Geometry check sheet. Reference: the model listing, model coordinates, mm. Face numbers are marked on the shaded views. A direction names the side the tool comes from. Give positions to 0.01 mm unless a question says otherwise; leave off trailing zeros. Put each result on its own line as item: value. Start each with the question number.
Q1. Go/stop test with flat-tipped pins: pin 1 (2 mm diameter, centred on y = -6.5, z = 1, fed in from -X); pin 2 (9.5 mm diameter, centred on y = -3, z = 37, fed in from -X); pin 3 (5 mm diameter, centred on x = 19, z = 4, fed in from -Y) (3 decimals). Record where each tip stops, or that it passes through.
Q2. Mould release check, pull along Y, two halves, no side actions. Record for the marked faces 5, 6 and 7: +Y half, -Y half, draft (parallel to the pull), parting line (faces both ways), or undercut.
Q3. Access from +Z, -Z, +X, -X, +Y, -Y to the whole of each face (thin tool, end or side, straight path). Record for the marked faces 1, 2, 3 and 4.
Q4. Material ranges on L1, parallel to Z at x = 0, y = 1.6; L2, parallel to X at y = 2.45, z = 0; L3, parallel to Y at x = -10.5, z = 40 (3 decimals), recorded low to high.
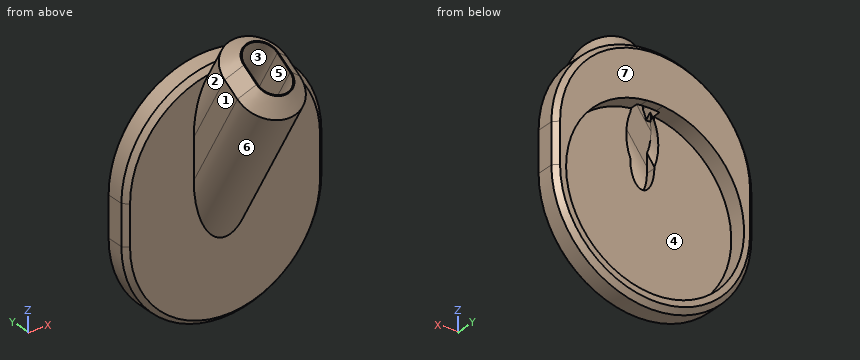
```python
from build123d import *

# Parameters (mm, degrees)
BOSS_EXTRUDE1_DEPTH     = 5.5
BOSS_EXTRUDE2_START     = -3.175
BOSS_EXTRUDE2_DEPTH     = 3.175
BOSS_EXTRUDE4_REACH     = 95.106
CUT_EXTRUDE1_DEPTH      = 2.54
CUT_EXTRUDE1_DEPTH_BACK = 12.7
CUT_EXTRUDE2_REACH      = 73.925
SKETCH7_R               = 5.08
CUT_EXTRUDE4_DEPTH      = 19.05
CHAMFER3_SIZE           = 4.445
CHAMFER4_SIZE           = 1.5875


with BuildPart() as part:
    # Sketch1 → Boss-Extrude1 (new body)
    # profile 1 of 2: a face of its own
    with BuildSketch(Plane(origin=(0, 0, 0), x_dir=(1, 0, 0), z_dir=(0, 1, 0))):
        with BuildLine():
            Line((31.75, -12.7), (31.75, 0))
            ThreePointArc((31.75, 0), (0, 31.75), (-31.75, 0))
            Line((-31.75, 0), (-31.75, -12.7))
            ThreePointArc((-31.75, -12.7), (0, -44.45), (31.75, -12.7))
        make_face()
        with BuildLine():
            ThreePointArc((2.5, -40.108217228), (0, -42.608217228), (-2.5, -40.108217228))
            Line((-2.5, -40.108217228), (-2.5, -28.139163101))
            ThreePointArc((-2.5, -28.139163101), (-19.071411851, 20.840915287), (28.25, 0))
            ThreePointArc((28.25, 0), (20.840915287, -19.071411851), (2.5, -28.139163101))
            Line((2.5, -28.139163101), (2.5, -40.108217228))
        make_face(mode=Mode.SUBTRACT)
    # profile 2 of 2: a face of its own
    with BuildSketch(Plane(origin=(0, 0, 0), x_dir=(1, 0, 0), z_dir=(0, 1, 0))):
        with BuildLine():
            Line((-2.5, -28.139163101), (-2.5, -40.108217228))
            ThreePointArc((-2.5, -40.108217228), (0, -42.608217228), (2.5, -40.108217228))
            Line((2.5, -40.108217228), (2.5, -28.139163101))
            ThreePointArc((2.5, -28.139163101), (0, -28.25), (-2.5, -28.139163101))
        make_face()
    extrude(amount=BOSS_EXTRUDE1_DEPTH)

    # Sketch1<3> → Boss-Extrude2 (add)
    with BuildSketch(Plane(origin=(0, 0, 0), x_dir=(1, 0, 0), z_dir=(0, 1, 0)).offset(BOSS_EXTRUDE2_START)):
        with BuildLine():
            Line((31.75, 0), (31.75, -12.7))
            ThreePointArc((31.75, -12.7), (0, -44.45), (-31.75, -12.7))
            Line((-31.75, -12.7), (-31.75, 0))
            ThreePointArc((-31.75, 0), (0, 31.75), (31.75, 0))
        make_face()
    extrude(amount=BOSS_EXTRUDE2_DEPTH)

    # Sketch9 → Boss-Extrude4 (add, up to next)
    with BuildSketch(Plane(origin=(0, -18.686909051, 52.366675913), x_dir=(1, 0, 0), z_dir=(-1.7076979057767106e-15, 0.4999999999999981, -0.8660254037844397)), mode=Mode.PRIVATE) as boss_extrude4_sk1:
        with BuildLine():
            Line((9.9425, 6.35), (9.9425, 0))
            ThreePointArc((9.9425, 0), (0, -9.9425), (-9.9425, 0))
            Line((-9.9425, 0), (-9.9425, 6.35))
            ThreePointArc((-9.9425, 6.35), (0, 16.2925), (9.9425, 6.35))
        make_face()
        with BuildLine():
            Line((5.18, 6.35), (5.18, 0))
            ThreePointArc((5.18, 0), (0, -5.18), (-5.18, 0))
            Line((-5.18, 0), (-5.18, 6.35))
            ThreePointArc((-5.18, 6.35), (0, 11.53), (5.18, 6.35))
        make_face(mode=Mode.SUBTRACT)
    boss_extrude4_tool1 = extrude(boss_extrude4_sk1.sketch, amount=BOSS_EXTRUDE4_REACH, mode=Mode.PRIVATE) - part.part
    add(boss_extrude4_tool1.solids().sort_by_distance((-9.613306, -21.43654, 50.779176))[0])

    # Sketch1<5> → Cut-Extrude1 (cut, two sides: drawn at the far end of the back side and taken through both)
    with BuildSketch(Plane(origin=(0, 0, 0), x_dir=(1, 0, 0), z_dir=(0, 1, 0)).offset(-CUT_EXTRUDE1_DEPTH_BACK)):
        with BuildLine():
            Line((-2.5, -28.139163101), (-2.5, -40.108217228))
            ThreePointArc((-2.5, -40.108217228), (0, -42.608217228), (2.5, -40.108217228))
            Line((2.5, -40.108217228), (2.5, -28.139163101))
            ThreePointArc((2.5, -28.139163101), (0, -28.25), (-2.5, -28.139163101))
        make_face()
    extrude(amount=CUT_EXTRUDE1_DEPTH + CUT_EXTRUDE1_DEPTH_BACK, mode=Mode.SUBTRACT)

    # Cut-Extrude2: up to this face of the body (flat: up to its plane)
    cut_extrude2_end = Plane(part.part.faces().sort_by_distance((0, 2.54, 35.153591808))[0])
    # Sketch6 → Cut-Extrude2 (cut, up to the picked face)
    with BuildSketch(Plane.XZ.offset(3.175), mode=Mode.PRIVATE) as cut_extrude2_sk1:
        with BuildLine():
            Line((3.81, 12.799261314), (3.81, 25.499261314))
            add(Edge.make_bspline(
                [(3.81, 25.499261314), (3.81, 33.119261314), (0, 33.119261314), (-3.81, 33.119261314), (-3.81, 25.499261314)],
                knots=[4.71238898, 4.71238898, 4.71238898, 6.283185307, 6.283185307, 7.853981634, 7.853981634, 7.853981634], degree=2, weights=[1, 0.707106781, 1, 0.707106781, 1]))
            Line((-3.81, 25.499261314), (-3.81, 12.799261314))
            add(Edge.make_bspline(
                [(-3.81, 12.799261314), (-3.81, 5.179261314), (0, 5.179261314), (3.81, 5.179261314), (3.81, 12.799261314)],
                knots=[1.570796327, 1.570796327, 1.570796327, 3.141592654, 3.141592654, 4.71238898, 4.71238898, 4.71238898], degree=2, weights=[1, 0.707106781, 1, 0.707106781, 1]))
        make_face()
    cut_extrude2_tool1 = split(extrude(cut_extrude2_sk1.sketch, amount=-CUT_EXTRUDE2_REACH, mode=Mode.PRIVATE), bisect_by=cut_extrude2_end, keep=Keep.BOTH, mode=Mode.PRIVATE)
    add(cut_extrude2_tool1.solids().sort_by(Axis((0, -3.175, 19.149261), (0, 1, 0)))[0], mode=Mode.SUBTRACT)

    # Sketch7 → Cut-Extrude4 (cut)
    with BuildSketch(Plane(origin=(0, -3.534663089, 6.122216058), x_dir=(-1, 0, 0), z_dir=(-1.5543122344752196e-15, 0.49999999999999956, -0.8660254037844389))):
        with Locations((0, 10)):
            Circle(SKETCH7_R)
    extrude(amount=-CUT_EXTRUDE4_DEPTH, mode=Mode.SUBTRACT)

    # Chamfer3
    chamfer3_edges = [part.edges().sort_by_distance(p)[0] for p in [
        (-9.9425, -21.436539708, 50.779175913),
        (0, -32.796627942, 44.220425913),
        (0, -10.076451474, 57.337925913),
        (9.9425, -21.436539708, 50.779175913),
    ]]
    chamfer(chamfer3_edges, length=CHAMFER3_SIZE)

    # Chamfer4
    # the kernel refuses this chamfer: 1.5875 mm, written as the material it takes off along each edge
    with BuildSketch(Plane(origin=(0, -3.175, 12.7), x_dir=(0.025619349712622985, 0, 0.9996717705928794), z_dir=(0.9996717705928794, 0, -0.025619349712622985))) as chamfer4_piece_1_section:
        Polygon((31.75 - CHAMFER4_SIZE, 0), (31.75, -CHAMFER4_SIZE), (31.75, 0), align=None)
    chamfer4_piece_1 = revolve(axis=Axis((0, -3.175, 12.7), (0, -1, 0)), revolution_arc=91.468041234, mode=Mode.PRIVATE)
    chamfer4_piece_1 = chamfer4_piece_1 - Plane(origin=(0, -7.049278044, 32.20970773), x_dir=(1, 0, 0), z_dir=(1.7076979057767106e-15, -0.4999999999999981, 0.8660254037844397)) * Cylinder(9.9425, 127, mode=Mode.PRIVATE)
    add(chamfer4_piece_1, mode=Mode.SUBTRACT)
    with BuildSketch(Plane(origin=(31.75, -3.175, 0), x_dir=(-0.9996219169112966, -0.02749587661058651, 0), z_dir=(0, 0, 1)), Plane(origin=(-31.75, -3.175, 12.7), x_dir=(0.9996219169112966, -0.02749587661058651, 0), z_dir=(0, 0, -1))) as chamfer4_piece_2:
        Polygon((CHAMFER4_SIZE * 0.999621916911, -CHAMFER4_SIZE * 0.0274958766106), (-CHAMFER4_SIZE * 0.0274958766106, -CHAMFER4_SIZE * 0.999621916911), (0, 0), align=None)
    extrude(amount=12.7, mode=Mode.SUBTRACT)
    with BuildSketch(Plane(origin=(0, -3.175, 0), x_dir=(-1, 0, 0), z_dir=(0, 0, 1))) as chamfer4_piece_3:
        Polygon((31.75 - CHAMFER4_SIZE, 0), (31.75, -CHAMFER4_SIZE), (31.75, 0), align=None)
    revolve(axis=Axis((0, -3.175, 0), (0, -1, 0)), revolution_arc=180, mode=Mode.SUBTRACT)
    with BuildSketch(Plane(origin=(0, 5.5, 0), x_dir=(1, 0, 0), z_dir=(0, 0, 1))) as chamfer4_piece_4:
        Polygon((31.75, -CHAMFER4_SIZE), (31.75 - CHAMFER4_SIZE, 0), (31.75, 0), align=None)
    revolve(axis=Axis((0, 5.5, 0), (0, 1, 0)), revolution_arc=180, mode=Mode.SUBTRACT)
    with BuildSketch(Plane(origin=(-31.75, 5.5, 0), x_dir=(-0.027495876610585654, -0.9996219169112968, 0), z_dir=(0, 0, 1)), Plane(origin=(31.75, 5.5, 12.7), x_dir=(0.027495876610585654, -0.9996219169112968, 0), z_dir=(0, 0, -1))) as chamfer4_piece_5:
        Polygon((CHAMFER4_SIZE * 0.999621916911, CHAMFER4_SIZE * 0.0274958766106), (-CHAMFER4_SIZE * 0.0274958766106, CHAMFER4_SIZE * 0.999621916911), (0, 0), align=None)
    extrude(amount=12.7, mode=Mode.SUBTRACT)
    with BuildSketch(Plane(origin=(0, 5.5, 12.7), x_dir=(-1, 0, 0), z_dir=(0, 0, -1))) as chamfer4_piece_6:
        Polygon((31.75, -CHAMFER4_SIZE), (31.75 - CHAMFER4_SIZE, 0), (31.75, 0), align=None)
    revolve(axis=Axis((0, 5.5, 12.7), (0, 1, 0)), revolution_arc=180, mode=Mode.SUBTRACT)
    with BuildSketch(Plane(origin=(0, -3.175, 12.7), x_dir=(1, 0, 0), z_dir=(0, 0, -1))) as chamfer4_piece_7_section:
        Polygon((31.75 - CHAMFER4_SIZE, 0), (31.75, -CHAMFER4_SIZE), (31.75, 0), align=None)
    chamfer4_piece_7 = revolve(axis=Axis((0, -3.175, 12.7), (0, -1, 0)), revolution_arc=91.468041234, mode=Mode.PRIVATE)
    chamfer4_piece_7 = chamfer4_piece_7 - Plane(origin=(0, -7.049278047, 32.209707734), x_dir=(1, 0, 0), z_dir=(1.7076979057767106e-15, -0.4999999999999981, 0.8660254037844397)) * Cylinder(9.9425, 127, mode=Mode.PRIVATE)
    add(chamfer4_piece_7, mode=Mode.SUBTRACT)


solid = part.part
```
Results found:
1. pin 1: stops at x = -6.19
1. pin 2: stops at x = -24.85
1. pin 3: stops at y = -3.175
2. face 5: undercut
2. face 6: -Y half
2. face 7: +Y half
3. face 1: +Z, -Z, -X, -Y
3. face 2: +Z
3. face 3: none
3. face 4: +Y
4. L1: z = -31.75 to -28.25, 42.61 to 44.45
4. L2: x = -31.75 to -28.25, 28.25 to 31.75
4. L3: y = -3.175 to 5.5
